Could you check a few things on this model? Use its own coordinates, in mm. Face numbers are marked on the shaded views. A direction names the side the tool comes from. Round coordinates to 2 decimals unless told otherwise and drop trailing zeros. Loops run counter-clockwise (first coordinate to the right, second up) from the corner with the lowest first, then second, coordinate; pieces in that order, holes last. Notation, with made-up numbers: (68, 46) - (116, 46) arc R18 ccw to (116, 81) - close; hole circle Ø4 at (37.5, 70). An arc over 180 degrees is marked (long way). Use one line per item in the form item = value.
```python
from build123d import *

# Parameters (mm, degrees)
SALIENTE_EXTRUIR1_DEPTH = 3
SALIENTE_EXTRUIR2_DEPTH = 130
CORTAR_EXTRUIR1_DEPTH   = 2
CORTAR_EXTRUIR2_DEPTH   = 29


with BuildPart() as part:
    # Croquis1 → Saliente-Extruir1 (new body)
    with BuildSketch(Plane.XY):
        Polygon((-180, 59.5), (-180, 66.5), (-173, 66.5), (173, 66.5), (180, 66.5), (180, 59.5), (180, -59.5), (180, -66.5), (173, -66.5), (-173, -66.5), (-180, -66.5), (-180, -59.5), align=None)
        with BuildLine():
            Line((-86.752968629, 57.900573009), (86.752968629, 57.900573009))
            ThreePointArc((86.752968629, 57.900573009), (100.895104253, 52.042708633), (106.752968629, 37.900573009))
            Line((106.752968629, 37.900573009), (106.752968629, -37.900573009))
            ThreePointArc((106.752968629, -37.900573009), (100.895104253, -52.042708633), (86.752968629, -57.900573009))
            Line((86.752968629, -57.900573009), (-86.752968629, -57.900573009))
            ThreePointArc((-86.752968629, -57.900573009), (-100.895104253, -52.042708633), (-106.752968629, -37.900573009))
            Line((-106.752968629, -37.900573009), (-106.752968629, 37.900573009))
            ThreePointArc((-106.752968629, 37.900573009), (-100.895104253, 52.042708633), (-86.752968629, 57.900573009))
        make_face(mode=Mode.SUBTRACT)
    extrude(amount=SALIENTE_EXTRUIR1_DEPTH)

    # Croquis2 → Saliente-Extruir2 (add)
    with BuildSketch(Plane.XY.offset(3)):
        with BuildLine():
            Line((-106.752968629, 37.900573009), (-106.752968629, -37.900573009))
            ThreePointArc((-106.752968629, -37.900573009), (-100.895104253, -52.042708633), (-86.752968629, -57.900573009))
            Line((-86.752968629, -57.900573009), (86.752968629, -57.900573009))
            ThreePointArc((86.752968629, -57.900573009), (100.895104253, -52.042708633), (106.752968629, -37.900573009))
            Line((106.752968629, -37.900573009), (106.752968629, 37.900573009))
            ThreePointArc((106.752968629, 37.900573009), (100.895104253, 52.042708633), (86.752968629, 57.900573009))
            Line((86.752968629, 57.900573009), (-86.752968629, 57.900573009))
            ThreePointArc((-86.752968629, 57.900573009), (-100.895104253, 52.042708633), (-106.752968629, 37.900573009))
        make_face()
    extrude(amount=-SALIENTE_EXTRUIR2_DEPTH)

    # Croquis3 → Cortar-Extruir1 (cut)
    with BuildSketch(Plane.XY.offset(3)):
        with BuildLine():
            Line((99.412909993, -57.909788035), (-99.412909993, -57.909788035))
            ThreePointArc((-99.412909993, -57.909788035), (-104.362657461, -55.859535503), (-106.412909993, -50.909788035))
            Line((-106.412909993, -50.909788035), (-106.412909993, 50.909788035))
            ThreePointArc((-106.412909993, 50.909788035), (-104.362657461, 55.859535503), (-99.412909993, 57.909788035))
            Line((-99.412909993, 57.909788035), (99.412909993, 57.909788035))
            ThreePointArc((99.412909993, 57.909788035), (104.362657461, 55.859535503), (106.412909993, 50.909788035))
            Line((106.412909993, 50.909788035), (106.412909993, -50.909788035))
            ThreePointArc((106.412909993, -50.909788035), (104.362657461, -55.859535503), (99.412909993, -57.909788035))
        make_face()
        with BuildLine():
            Line((-104.412909993, -50.909788035), (-104.412909993, 50.909788035))
            ThreePointArc((-104.412909993, 50.909788035), (-102.948443899, 54.445321941), (-99.412909993, 55.909788035))
            Line((-99.412909993, 55.909788035), (99.412909993, 55.909788035))
            ThreePointArc((99.412909993, 55.909788035), (102.948443899, 54.445321941), (104.412909993, 50.909788035))
            Line((104.412909993, 50.909788035), (104.412909993, -50.909788035))
            ThreePointArc((104.412909993, -50.909788035), (102.948443899, -54.445321941), (99.412909993, -55.909788035))
            Line((99.412909993, -55.909788035), (-99.412909993, -55.909788035))
            ThreePointArc((-99.412909993, -55.909788035), (-102.948443899, -54.445321941), (-104.412909993, -50.909788035))
        make_face(mode=Mode.SUBTRACT)
    extrude(amount=-CORTAR_EXTRUIR1_DEPTH, mode=Mode.SUBTRACT)

    # Croquis4 → Cortar-Extruir2 (cut)
    with BuildSketch(Plane.XY.offset(3)):
        with BuildLine():
            Line((-180, 40.936641428), (-172.017039574, 40.936641428))
            ThreePointArc((-172.017039574, 40.936641428), (-168.413104138, 37.332705992), (-172.017039574, 33.728770556))
            Line((-172.017039574, 33.728770556), (-180, 33.728770556))
            ThreePointArc((-180, 33.728770556), (-183.603935436, 37.332705992), (-180, 40.936641428))
        make_face()
        with BuildLine():
            Line((-180, -22.678860967), (-172.017039574, -22.678860967))
            ThreePointArc((-172.017039574, -22.678860967), (-168.533610515, -26.162290026), (-172.017039574, -29.645719085))
            Line((-172.017039574, -29.645719085), (-180, -29.645719085))
            ThreePointArc((-180, -29.645719085), (-183.483429059, -26.162290026), (-180, -22.678860967))
        make_face()
        with BuildLine():
            Line((180, 31.976759047), (168.655882601, 31.976759047))
            ThreePointArc((168.655882601, 31.976759047), (163.299935657, 37.332705992), (168.655882601, 42.688652937))
            Line((168.655882601, 42.688652937), (180, 42.688652937))
            ThreePointArc((180, 42.688652937), (185.355946945, 37.332705992), (180, 31.976759047))
        make_face()
        with BuildLine():
            Line((180, -31.731355776), (168.655882601, -31.731355776))
            ThreePointArc((168.655882601, -31.731355776), (163.086816851, -26.162290026), (168.655882601, -20.593224276))
            Line((168.655882601, -20.593224276), (180, -20.593224276))
            ThreePointArc((180, -20.593224276), (185.56906575, -26.162290026), (180, -31.731355776))
        make_face()
    extrude(amount=-CORTAR_EXTRUIR2_DEPTH, mode=Mode.SUBTRACT)


solid = part.part
```
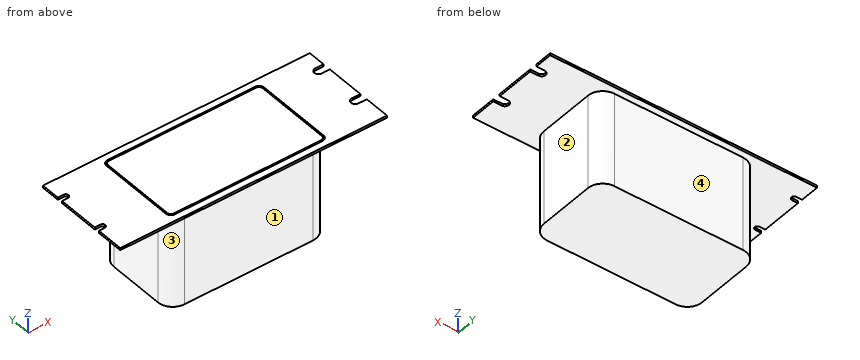
1. If we section it at B-B, the plane x = -36: Write out the boundary of the cut face in (y, z), plus the area to 3 significant figures.
Solution:
outline = (-66.5, 0) - (-57.9, 0) - (-57.9, -127) - (57.9, -127) - (57.9, 0) - (66.5, 0) - (66.5, 3) - (57.91, 3) - (57.91, 1) - (55.91, 1) - (55.91, 3) - (-55.91, 3) - (-55.91, 1) - (-57.91, 1) - (-57.91, 3) - (-66.5, 3) - close
area = 15,100 mm^2
2. On a 3-axis mill with a long thin cutter (end or side, diameter ignored), from which of +Z, -Z, +X, -X, +Y, -Y can I reach the whole of each face in a straight line? I mean the marked faces 1, 2, 3 and 4. Say none if no direction works.
Solution:
face_1 = -Z, +X, -X, -Y
face_2 = -Z, +X, +Y, -Y
face_3 = -Z, -X, -Y
face_4 = -Z, +X, -X, +Y
3. For P1, Ø3, axis at x = 28.5, z = -78, coming from the +Y side; P2, Ø3, axis at y = 48, z = -20, coming from the -X side; P3, Ø10, axis at y = 31, z = -33.5, coming from the -X side, each with a flat end and sliding along its axis, tell me the tip position at first contact or that it passes through.
Solution:
P1 = 57.9
P2 = -104.81
P3 = -106.75
4. Please list where these lines run through material, in increasing order: line 1 along X through (y, z) = (3, -99.5); line 2 along Y through (x, z) = (10, -27); line 3 along Z through (x, y) = (-147.5, 33.5).
Solution:
line_1 = -106.75 to 106.75
line_2 = -57.9 to 57.9
line_3 = 0 to 3
5. If we section it at D-D, the plane x = -111: Write out the boundary of the cut face in (y, z), plus the area to 3 significant figures.
Solution:
outline = (-66.5, 0) - (66.5, 0) - (66.5, 3) - (-66.5, 3) - close
area = 399 mm^2
6. If we section it at A-A, the plane y = 22: Write out the boundary of the cut face in (x, z), plus the area to 3 significant figures.
Solution:
outline = (-180, 0) - (-106.75, 0) - (-106.75, -127) - (106.75, -127) - (106.75, 0) - (180, 0) - (180, 3) - (106.41, 3) - (106.41, 1) - (104.41, 1) - (104.41, 3) - (-104.41, 3) - (-104.41, 1) - (-106.41, 1) - (-106.41, 3) - (-180, 3) - close
area = 28,200 mm^2
7. If we section it at C-C, the plane z = -101.5: Write out the boundary of the cut face in (x, y), plus the area to 3 significant figures.
Solution:
outline = (-106.75, -37.9) arc R20 ccw to (-86.75, -57.9) - (86.75, -57.9) arc R20 ccw to (106.75, -37.9) - (106.75, 37.9) arc R20 ccw to (86.75, 57.9) - (-86.75, 57.9) arc R20 ccw to (-106.75, 37.9) - close
area = 24,400 mm^2
